Can you work these out from the model? Positions are in its coordinate system, mm. A direction names the side the tool comes from. Give positions to 0.01 mm unless a question says otherwise; leave off trailing zeros. Order: outer loops, then holes, each group sorted by start corner. A loop starts at its lowest first (then second) coordinate and runs counter-clockwise, first axis right, second up. Notation, with made-up numbers: M 43.5,82 L 97.5,82 A16 cw 97.5,95 Z; hole C -26.5,5.25 d8. An arc over 180 degrees is marked long. Use one line per item in the form item = value. Start each with the question number.
1. I want a section at A-A, the plane y = -170. List the corners of the cut face in (x, z) for me.
2. Will these pins go through, and if not, where does the flat tip stop? P1, Ø3, axis at x = 37.5, y = -41.5, coming from the +Z side; P2, Ø0.5, axis at y = -116, z = 0.5, coming from the -X side; P3, Ø1.1, axis at x = 55, z = 0.5, coming from the -Y side.
3. I want a section at D-D, the plane y = -99.5. List the corners of the cut face in (x, z) for me, and give its area (3 significant figures).
4. I need wall thicknesses on L1, parallel to Z at x = 54.5, y = -32.5; L2, parallel to X at y = -128, z = 2.2; L3, parallel to Y at x = 49.5, z = 0.65. Which ranges of each line are inside material? Lowest first, please.
5. I want a section at C-C, the plane x = 49.5. List the corners of the cut face in (y, z) for me, and give its area (3 significant figures).
6. For faces 1 (the face through (35.5, -111, 2)), 2 (the face through (34.5, -109, 2)), 3 (the face through (35, -43.5, 2.5)), which set-ups out of +Z, -Z, +X, -X, +Y, -Y let a thin tool reach every point of the face, with its end or its side?
7. I want a section at B-B, the plane z = 1.75. List the corners of the cut face in (x, y) for me, and give its area (3 significant figures).
```python
from build123d import *

# Parameters (mm, degrees)
PAD_DEPTH       = 1
PAD001_DEPTH    = 3
POCKET_DEPTH    = 35.501
POCKET001_DEPTH = 35.501


with BuildPart() as part:
    # Sketch → Pad (new body)
    with BuildSketch(Plane.XY):
        with BuildLine():
            Line((7, 0), (63, 0))
            ThreePointArc((70, -7), (67.949747, -2.050253), (63, 0))
            Line((70, -7), (70, -33))
            ThreePointArc((63, -40), (67.949747, -37.949747), (70, -33))
            Line((63, -40), (47, -40))
            ThreePointArc((47, -40), (42.050253, -42.050253), (40, -47))
            Line((40, -47), (40, -160))
            Line((36, -180), (40, -160))
            ThreePointArc((34, -180), (35, -180.819804), (36, -180))
            Line((30, -160), (34, -180))
            Line((30, -47), (30, -160))
            ThreePointArc((30, -47), (27.949747, -42.050253), (23, -40))
            Line((23, -40), (7, -40))
            ThreePointArc((0, -33), (2.050253, -37.949747), (7, -40))
            Line((0, -33), (0, -7))
            ThreePointArc((7, 0), (2.050253, -2.050253), (0, -7))
        make_face()
    extrude(amount=PAD_DEPTH)

    # Sketch001 (on Face18 of Pad) → Pad001 (join)
    with BuildSketch(Plane.XY.offset(1)):
        Polygon((34.5, -180), (35.5, -180), (35.5, -160), (35.5, -47), (35.5, -40), (34.5, -40), (34.5, -47), (34.5, -160), align=None)
    extrude(amount=PAD001_DEPTH)

    # Sketch002 (on Face26 of Pad001) → Pocket (cut, through all)
    with BuildSketch(Plane(origin=(34.5, 0, 0), x_dir=(0, -1, 0), z_dir=(-1, 0, 0))):
        Polygon((160, 4), (180, 1), (180, 4), align=None)
    extrude(amount=-POCKET_DEPTH, mode=Mode.SUBTRACT)

    # Sketch003 (on Face22 of Pocket) → Pocket001 (cut, through all)
    with BuildSketch(Plane(origin=(34.5, 0, 0), x_dir=(0, -1, 0), z_dir=(-1, 0, 0))):
        Polygon((40, 1), (40, 4), (47, 4), align=None)
    extrude(amount=-POCKET001_DEPTH, mode=Mode.SUBTRACT)


solid = part.part
```
Check result:
q1.outline = M 32,0 L 38,0 L 38,1 L 35.5,1 L 35.5,2.5 L 34.5,2.5 L 34.5,1 L 32,1 Z
q2.P1 = 1
q2.P2 = 30
q2.P3 = -40
q3.outline = M 30,0 L 40,0 L 40,1 L 35.5,1 L 35.5,4 L 34.5,4 L 34.5,1 L 30,1 Z
q3.area = 13.0 mm2
q4.L1 = 0 to 1
q4.L2 = 34.5 to 35.5
q4.L3 = -40 to 0
q5.outline = M -40,0 L 0,0 L 0,1 L -40,1 Z
q5.area = 40.0 mm2
q6.face_1 = +Z, +X, +Y, -Y
q6.face_2 = +Z, -X, +Y, -Y
q6.face_3 = +Z, +X, -X, +Y
q7.outline = M 34.5,-175 L 35.5,-175 L 35.5,-41.75 L 34.5,-41.75 Z
q7.area = 133 mm2
